Can you work these out from the model? Positions are in its coordinate system, mm. A direction names the side the tool comes from. Round coordinates to 2 decimals unless told otherwise and drop trailing zeros. Order: outer loops, then holes, each group sorted by start corner. A loop starts at its lowest first (then second) coordinate and runs counter-clockwise, first axis right, second up. Notation, with made-up numbers: (47, 0) - (92, 0) arc R17 cw to (92, 22) - close; hole circle Ø6 at (-36, -7). An arc over 180 degrees is marked (long way). Write item = value, one per line.
Autodesk Inventor part; units mm, degrees
ref_plane "Work Plane1" through (1.525, 0, 0) normal (0, 0, 1) x (1, 0, 0)
ref_plane "YZ Plane" through (0, 0, 0) normal (1, 0, 0) x (0, 1, 0)
ref_plane "XZ Plane" through (0, 0, 0) normal (0, 1, 0) x (-1, 0, 0)
sketch "Sketch1" plane through (0, 0, 0) normal (0, 0, 1) x (1, 0, 0)
  line L0 (0, 7.315) -> (0, 5)
  line L1 (74, 5) -> (100, 5)
  line L2 (100, 5) -> (100, 0)
  line L3 (100, 0) -> (-0.6001, 0)
  line L4 (-20.7201, 0) -> (120.12, 0)
  line L5 (-0.6001, 0) -> (-0.6001, 7.315)
  line L6 (-0.6001, 7.315) -> (0, 7.315)
  line L7 (74, 5) -> (73.0797, 5)
  line L8 (73.0797, 5) -> (0, 5)
  line L9 (0, -1.463) -> (0, 8.778)
  dimension "d0" = 100
  dimension "d1" = 26
  dimension "d2" = 10
  dimension "d9" = 0.6001
  dimension "d10" = 14.63
  dimension "d13" = 0.9203
  dimension "d14" = 10
revolve "Body" add sketch "Sketch1" angle 360 about axis through (100, 0, 0) along (-1, 0, 0)
sketch "Sketch2" plane through (-0.6001, 0, 0) normal (-1, 0, 0) x (0, 0, 1)
  line L0 (0, 9.2376) -> (8, 4.6188)
  line L1 (8, 4.6188) -> (8, -4.6188)
  line L2 (8, -4.6188) -> (0, -9.2376)
  line L3 (0, -9.2376) -> (-8, -4.6188)
  line L4 (-8, -4.6188) -> (-8, 4.6188)
  line L5 (-8, 4.6188) -> (0, 9.2376)
  point P0 (0, 0)
  point P1 (0, 0)
  dimension "d11" = 16
extrude "Head" add sketch "Sketch2" along normal blind 5.8
sketch "Sketch4" plane through (0, 0, 0) normal (0, 0, 1) x (1, 0, 0)
  line L0 (-6.4001, 8) -> (-6.4001, 9.2376)
  line L1 (-6.4001, 9.2376) -> (-5.6856, 9.2376)
  line L2 (-5.6856, 9.2376) -> (-6.4001, 8)
  line L3 (-7.5601, 0) -> (0.5599, 0)
  line L4 (-0.6001, 9.2376) -> (-6.4001, 9.2376)
  line L5 (-6.4001, 4.6188) -> (-6.4001, 9.2376)
  dimension "d5" = 30
  dimension "d19" = 16
revolve "Chamfer1" cut sketch "Sketch4" angle 360 about axis through (-10, 0, 0) along (1, 0, 0)
thread "Thread"
chamfer "Chamfer2" distance 0.9202 distance2 0.9203 1 edges at (100, -5, 0) measured on face at (100, 1.175, -0.5081)
ref_plane "Work Plane1" through (1.525, 0, 0) normal (0, 0, 1) x (1, 0, 0)
equation "\"d11\" = SW"
equation "\"d3\" = KOH - SD"
equation "\"d15\" = GEL"
equation "\"d6\" = -0.5 * SPD + 0.5 * GD"
equation "\"d0\" = NLG"
equation "\"d1\" = GEL"
equation "\"d2\" = GD"
equation "\"d10\" = SD2"
equation "\"d14\" = BDM"
equation "\"d5\" = ANG1"
equation "\"d19\" = SW0"
equation "\"NLG\" = 100"
equation "\"GD\" = NND"
equation "\"BDM\" = NND"
equation "\"KOH\" = 6.4"
equation "\"GEL\" = 26"
equation "\"SW\" = 16"
equation "\"SW0\" = SW"
equation "\"SPD\" = NND - 1.2269 * PTC"
equation "\"SD2\" = 14.63"
equation "\"SD\" = 0.6"
equation "\"ANG1\" = 30deg"
equation "\"GAL\" = 0.61345 * PTC"
equation "\"GUL\" = 0.61345 * PTC"
equation "\"RR\" = 0.4"
equation "\"GD1\" = THREADDIA - 1.2269 * PTC"
equation "\"SDH\" = SD2"
equation "\"TOA\" = 30deg"
equation "\"PTC\" = 1.5"
equation "\"E0\" = 1.155 * SW"
properties part number "ISO 4014 - M10 x 100" material "Stainless Steel, 440C"
(1) If I drill on line 1 (Y direction, x = 26, z = 3); line 2 (X direction, y = -6, z = 5.25), over which ranges is the centre line in solid material (lowest first)? Write a range as from..to.
Computed:
line_1 = -4..4
line_2 = -6.4..-0.6
(2) Will these pins go through, and if not, where does the flat tip stop? P1, Ø1.5, axis at x = 69.5, z = -4.5, coming from the -Y side; P2, Ø2, axis at x = 30, z = -2.5, coming from the +Y side; P3, Ø5, axis at x = 49, y = 0, coming from the +Z side.
Computed:
P1 = -3.31
P2 = 4.77
P3 = 5
(3) If we section it at A-A (x = 75): Write out the boundary of the cut face in (y, z).
Computed:
outline = circle Ø10 at (0, 0)
(4) On a 3-axis mill with a long thin cutter (end or side, diameter ignored), from which of +Z, -Z, +X, -X, +Y, -Y can I reach the whole of each face in a straight line? I mean faces 1 (the face through (-6.226, -8.301, 0.02)), 2 (the face through (0, 5, 2)). Say none if no direction works.
Computed:
face_1 = -X, -Y
face_2 = +X
